Part model, mm, in its own coordinate system. Round coordinates to 2 decimals unless told otherwise and drop trailing zeros. Loops run counter-clockwise (first coordinate to the right, second up) from the corner with the lowest first, then second, coordinate; pieces in that order, holes last.
(1) Cut at A-A on z = 12.5. List the corners of the cut face in (x, y), then the cut area to 3 significant figures.
(2) Cut at B-B on x = -51. List the corners of the cut face in (y, z), then the cut area to 3 significant figures.
(3) Cut at C-C on y = -159.5. List the corners of the cut face in (x, z), then the cut area to 3 significant figures.
(4) Probe probe 1 along Y at (x, z) = (-13, 7.25); probe 2 along X at (y, z) = (184, 2.5); probe 3 along Y at (x, z) = (390.5, 13.5). List the from-to ranges inside material, lowest first.
(5) Flat gauge pins, fed straight in: pin 1 (5.5 mm diameter, centred on y = -203, z = 9, fed in from +X); pin 2 (5.5 mm diameter, centred on x = -423.5, z = 7, fed in from -Y); pin 3 (5.5 mm diameter, centred on y = 14, z = 6, fed in from -X). Where does each tip first touch, or does it go through?
from build123d import *

# Parameters (mm, degrees)
F0_W     = 19.05
F0_H     = 25.4
F1_DEPTH = 19.05


with BuildPart() as f1:
    # F0 (on Top) → F1 (new body)
    with BuildSketch(Plane.XY):
        with BuildLine():
            Line((414.764641, 224.573665), (-410.735359, 224.573665))
            Line((-410.735359, 224.573665), (-410.735359, 154.723665))
            Line((-410.735359, 154.723665), (-410.735359, 129.323665))
            Line((-410.735359, 129.323665), (-410.735359, -105.626335))
            Line((-410.735359, -105.626335), (-410.735359, -131.026335))
            Line((-410.735359, -131.026335), (-410.735359, -385.026335))
            ThreePointArc((-410.735359, -385.026335), (-395.856384, -420.94736), (-359.935359, -435.826335))
            Line((-359.935359, -435.826335), (363.964641, -435.826335))
            ThreePointArc((363.964641, -435.826335), (399.885665, -420.94736), (414.764641, -385.026335))
            Line((414.764641, -385.026335), (414.764641, -131.026335))
            Line((414.764641, -131.026335), (414.764641, -105.626335))
            Line((414.764641, -105.626335), (414.764641, 129.323665))
            Line((414.764641, 129.323665), (414.764641, 154.723665))
            Line((414.764641, 154.723665), (414.764641, 224.573665))
        make_face()
        with BuildLine():
            Line((90.914641, -397.726335), (-86.885359, -397.726335))
            ThreePointArc((-86.885359, -397.726335), (-95.865615, -394.006591), (-99.585359, -385.026335))
            ThreePointArc((-99.585359, -385.026335), (-95.865615, -376.046079), (-86.885359, -372.326335))
            Line((-86.885359, -372.326335), (90.914641, -372.326335))
            ThreePointArc((90.914641, -372.326335), (99.894897, -376.046079), (103.614641, -385.026335))
            ThreePointArc((103.614641, -385.026335), (99.894897, -394.006591), (90.914641, -397.726335))
        make_face(mode=Mode.SUBTRACT)
        with Locations((-420.260359, 142.023665)):
            Rectangle(F0_W, F0_H)
        with Locations((424.289641, 142.023665)):
            Rectangle(F0_W, F0_H)
        with Locations((-420.260359, -118.326335)):
            Rectangle(F0_W, F0_H)
        with Locations((424.289641, -118.326335)):
            Rectangle(F0_W, F0_H)
    extrude(amount=F1_DEPTH)


solid = f1.part
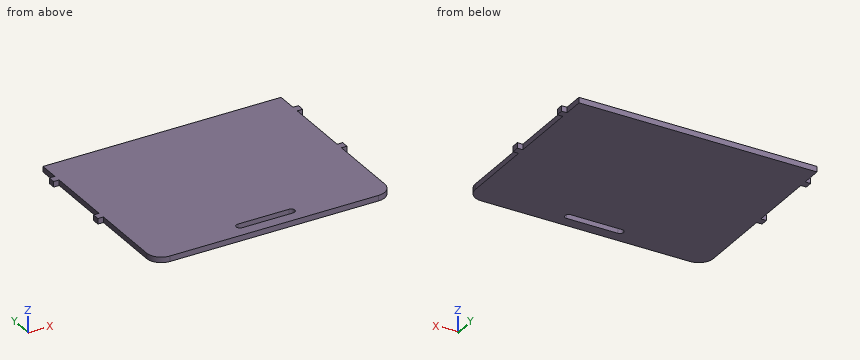
Final values:
1. outline: (-429.79, -131.03) - (-410.74, -131.03) - (-410.74, -385.03) arc R50.8 ccw to (-359.94, -435.83) - (363.96, -435.83) arc R50.8 ccw to (414.76, -385.03) - (414.76, -131.03) - (433.81, -131.03) - (433.81, -105.63) - (414.76, -105.63) - (414.76, 129.32) - (433.81, 129.32) - (433.81, 154.72) - (414.76, 154.72) - (414.76, 224.57) - (-410.74, 224.57) - (-410.74, 154.72) - (-429.79, 154.72) - (-429.79, 129.32) - (-410.74, 129.32) - (-410.74, -105.63) - (-429.79, -105.63) - close; hole (-86.89, -397.73) - (90.91, -397.73) arc R12.7 ccw to (90.91, -372.33) - (-86.89, -372.33) arc R12.7 ccw to start
1. area: 541,000 mm2
2. outline: (-435.83, 0) - (-397.73, 0) - (-397.73, 19.05) - (-435.83, 19.05) - close; (-372.33, 0) - (224.57, 0) - (224.57, 19.05) - (-372.33, 19.05) - close
2. area: 12,100 mm2
3. outline: (-410.74, 0) - (414.76, 0) - (414.76, 19.05) - (-410.74, 19.05) - close
3. area: 15,700 mm2
4. probe 1: y = -435.83 to -397.73, -372.33 to 224.57
4. probe 2: x = -410.74 to 414.76
4. probe 3: y = -428.35 to 224.57
5. pin 1: stops at x = 414.76
5. pin 2: stops at y = -131.03
5. pin 3: stops at x = -410.74
